```python
from build123d import *

# Parameters (mm, degrees)
F0_W     = 8.6868
F0_H     = 1.27
F1_DEPTH = 1.27
F2_W     = 20.828
F2_H     = 1.778
F3_DEPTH = 1.778
F4_W     = 15.24
F4_H     = 1.27
F5_DEPTH = 1.27


with BuildPart() as f1:
    # F0 (on Top) → F1 (new body)
    with BuildSketch(Plane.XY):
        Polygon((-4.3434, 6.983239), (-5.6134, 6.983239), (-5.6134, -43.816761), (-4.3434, -43.816761), (-4.3434, -41.276761), (-4.3434, -40.006761), (-4.3434, -34.926761), (-4.3434, -33.656761), align=None)
        with Locations((0, -34.291761)):
            Rectangle(F0_W, F0_H)
        Polygon((4.3434, 6.983239), (4.3434, -33.656761), (4.3434, -34.926761), (4.3434, -40.006761), (4.3434, -41.276761), (4.3434, -43.816761), (5.6134, -43.816761), (5.6134, 6.983239), align=None)
        with Locations((0, -40.641761)):
            Rectangle(F0_W, F0_H)
    extrude(amount=F1_DEPTH)

    # F2 (on face) → F3 (join)
    with BuildSketch(Plane.XY.offset(1.27)):
        with Locations((0, -6.605761)):
            Rectangle(F2_W, F2_H)
    extrude(amount=F3_DEPTH)

    # F4 (on face) → F5 (join)
    with BuildSketch(Plane.XY.offset(1.27)):
        with Locations((0, -29.099032)):
            Rectangle(F4_W, F4_H)
    extrude(amount=F5_DEPTH)


solid = f1.part
```
Geometry: final body of the model. Coordinates: model frame, mm. A direction names the side the tool comes from. Round coordinates to 2 decimals unless told otherwise and drop trailing zeros. Order: outer loops, then holes, each group sorted by start corner. A loop starts at its lowest first (then second) coordinate and runs counter-clockwise, first axis right, second up. Notation, with made-up numbers: M 15,-1 L 24,-1 A24 ccw 24,35 Z; hole C 20,-9 d4. An arc over 180 degrees is marked long. Use one line per item in the form item = value. Start each with the question number.
Q1. Pin query (flat end, axial travel): pin 1 Ø1.4 at (x, y) = (-5, -1.5) entering from +Z; pin 2 Ø1.4 at (x, z) = (2.5, 2) entering from -Y; pin 3 Ø1 at (y, z) = (-42.5, 0.5) entering from +X. Return the tip coordinate at first contact, or that it passes through.
Q2. Mould query, pull axis X, two halves, no side actions, for faces 4 (the face through (-7.62, -29, 2)), 5 (the face through (0, -29, 1.27)), 6 (the face through (0, -29.734, 2)). Classes: +X half, -X half, draft (parallel to the pull), parting line (faces both ways), or undercut.
Q3. Cut plane C-C (z = 0.8). Return loops of the section in (x, y), and give its area (3 significant figures).
Q4. Cut plane D-D (x = 3.5). Return loops of the section in (y, z), and give its area (3 significant figures).
Q5. Material intervals for line 1 (X direction, y = -36, z = 1.2); line 2 (Y direction, x = 1.25, z = 1.15); line 3 (Y direction, x = -4, z = 2.2), sorted ascending. Write a range as [from, to].
Q6. Cut plane A-A (x = -6.75). Return loops of the section in (y, z).
Q7. Cut plane B-B (y = -19). Return loops of the section in (x, z), and give its area (3 significant figures).
Q8. Access query for faces 1 (the face through (0, -29, 2.54)), 2 (the face through (8, -7, 1.27)), 3 (the face through (0, -40.007, 1)). Directions: +Z, -Z, +X, -X, +Y, -Y. A direction counts if a zero-diameter tool reaches every point of the face in a straight line with its end or side. Return the directions, or none.
Geometry results:
q1.pin_1 = 1.27
q1.pin_2 = -29.73
q1.pin_3 = 5.61
q2.face_4 = -X half
q2.face_5 = undercut
q2.face_6 = draft
q3.outline = M -5.61,-43.82 L -4.34,-43.82 L -4.34,-41.28 L 4.34,-41.28 L 4.34,-43.82 L 5.61,-43.82 L 5.61,6.98 L 4.34,6.98 L 4.34,-33.66 L -4.34,-33.66 L -4.34,6.98 L -5.61,6.98 Z; hole M -4.34,-40.01 L 4.34,-40.01 L 4.34,-34.93 L -4.34,-34.93 Z
q3.area = 151 mm^2
q4.outline = M -41.28,0 L -40.01,0 L -40.01,1.27 L -41.28,1.27 Z; M -34.93,0 L -33.66,0 L -33.66,1.27 L -34.93,1.27 Z; M -29.73,1.27 L -28.46,1.27 L -28.46,2.54 L -29.73,2.54 Z; M -7.49,1.27 L -5.72,1.27 L -5.72,3.05 L -7.49,3.05 Z
q4.area = 8.00 mm^2
q5.line_1 = [-5.61, -4.34], [4.34, 5.61]
q5.line_2 = [-41.28, -40.01], [-34.93, -33.66]
q5.line_3 = [-29.73, -28.46], [-7.49, -5.72]
q6.outline = M -29.73,1.27 L -28.46,1.27 L -28.46,2.54 L -29.73,2.54 Z; M -7.49,1.27 L -5.72,1.27 L -5.72,3.05 L -7.49,3.05 Z
q7.outline = M -5.61,0 L -4.34,0 L -4.34,1.27 L -5.61,1.27 Z; M 4.34,0 L 5.61,0 L 5.61,1.27 L 4.34,1.27 Z
q7.area = 3.23 mm^2
q8.face_1 = +Z, +X, -X, -Y
q8.face_2 = -Z, +X, +Y, -Y
q8.face_3 = +Z, -Z
